For this review, take the finished solid that the model builds, in its own axes (mm). A direction names the side the tool comes from. Round coordinates to 2 decimals unless told otherwise and drop trailing zeros. Order: outer loops, then holes, each group sorted by start corner. A loop starts at its lowest first (then second) coordinate and runs counter-clockwise, first axis right, second up.
from build123d import *

# Parameters (mm, degrees)
F1_DEPTH = 63.5
F0_W     = 4.3192696064
F0_H     = 12.0912648122
F0_H_2   = 11.3655438513
F0_H_3   = 5.1181913365
F2_DEPTH = 25.4
F3_DEPTH = 7.9375
F5_R     = 6.35


with BuildPart() as f1:
    # F0 (on Front) → F1 (new body, symmetric)
    with BuildSketch(Plane.XZ):
        Polygon((-41.275, -9.525), (41.275, -9.525), (41.275, 9.525), (29.9094561487, 9.525), (-41.275, 9.525), align=None)
    extrude(amount=F1_DEPTH, both=True)

    # F0 (on Front) → F2 (join, symmetric)
    with BuildSketch(Plane.XZ):
        with BuildLine():
            Line((29.9094561487, 9.525), (41.275, 9.525))
            Line((41.275, 9.525), (41.275, 37.4912648122))
            ThreePointArc((41.275, 37.4912648122), (45.9246798487, 48.7165849636), (57.15, 53.3662648122))
            Line((57.15, 53.3662648122), (84.2568697843, 53.3662648122))
            Line((84.2568697843, 53.3662648122), (84.2568697843, 64.7318086635))
            Line((84.2568697843, 64.7318086635), (78.3901438117, 64.7318086635))
            Line((78.3901438117, 64.7318086635), (57.15, 64.7318086635))
            ThreePointArc((57.15, 64.7318086635), (37.8880267196, 56.7532380926), (29.9094561487, 37.4912648122))
            Line((29.9094561487, 37.4912648122), (29.9094561487, 9.525))
        make_face()
        with Locations((86.4165045875, 47.3206324061)):
            Rectangle(F0_W, F0_H)
        with Locations((86.4165045875, 59.0490367378)):
            Rectangle(F0_W, F0_H_2)
        with Locations((86.4165045875, 67.2909043317)):
            Rectangle(F0_W, F0_H_3)
        Polygon((88.5761393907, 69.85), (88.5761393907, 64.7318086635), (88.5761393907, 53.3662648122), (88.5761393907, 41.275), (135.0568697843, 41.275), (135.0568697843, 69.85), align=None)
    extrude(amount=F2_DEPTH, both=True)

    # F0 (on Front) → F3 (join, symmetric)
    with BuildSketch(Plane.XZ):
        with BuildLine():
            add(Edge.make_bspline(
                [(-41.275, 9.525), (-36.5560054779, 38.5108739138), (-31.082380563, 73.5029876232), (78.3901438117, 64.7318086635)],
                knots=[0, 0, 0, 0, 131.7859566353, 131.7859566353, 131.7859566353, 131.7859566353], degree=3))
            Line((-41.275, 9.525), (29.9094561487, 9.525))
            Line((29.9094561487, 9.525), (29.9094561487, 37.4912648122))
            ThreePointArc((29.9094561487, 37.4912648122), (37.8880267196, 56.7532380926), (57.15, 64.7318086635))
            Line((57.15, 64.7318086635), (78.3901438117, 64.7318086635))
        make_face()
    extrude(amount=F3_DEPTH, both=True)

    # F0 (on Front) → F4 (revolve)
    with BuildSketch(Plane.XZ):
        Polygon((88.5761393907, 69.85), (88.5761393907, 64.7318086635), (88.5761393907, 53.3662648122), (88.5761393907, 41.275), (135.0568697843, 41.275), (135.0568697843, 69.85), align=None)
    revolve(axis=Axis((135.0568697843, 0, 55.5625), (0, 0, 1)))

    # F5
    f5_edges = [f1.edges().sort_by_distance(p)[0] for p in [
        (41.275, -63.5, 0),
        (-41.275, -63.5, 0),
        (41.275, 63.5, 0),
        (-41.275, 63.5, 0),
    ]]
    fillet(f5_edges, radius=F5_R)


solid = f1.part
(1) Add section B-B on y = 39.5. Give the boundary of the cut face in (x, z) (3 decimals), plus the area to 3 significant figures.
(2) Tool access review of faces 1 (the face through (134, -1, 41.275)), 2 (the face through (55, 25.4, 54)), 3 (the face through (29.909, -17, 24)): name each direction out of +Z, -Z, +X, -X, +Y, -Y from which nothing blocks a thin tool from reaching the whole face with its end or side.
(3) Clearance check with flat-ended pins moving along their axes: P1, Ø10, axis at y = 12.5, z = 7, coming from the +X side (3 decimals); P2, Ø14, axis at y = 20.5, z = 29.5, coming from the -X side; P3, Ø1.5, axis at x = 144.5, z = 61.5, coming from the +Y side; P4, Ø18, axis at x = 74, z = 30, coming from the +Y side. State where each tip first meets the part, or that it passes through.
(4) Add section C-C on x = 150.5. Give the boundary of the cut face in (y, z) (3 decimals), plus the area to 3 significant figures.
(5) Add section A-A on z = -1. Give the boundary of the cut face in (x, y) (3 decimals).
(6) Draft analysis for pull direction X (two halves, no side actions). For faces 4 (the face through (-39.365, 61.689, -0.133)), 5 (the face through (55, -25.4, 54)), 6 (the face through (71, 0, 53.366)), state which applies: pulls with the +X half, pulls with the -X half, needs draft (parallel to the pull), parting line crosses it, or undercut.
(7) Wall thickness on L1, parallel to Y at x = 25, z = 56; L2, parallel to Z at x = -4.5, y = 31 (3 decimals); L3, parallel to X at y = 26, z = 3 (3 decimals): over which ranges is each line inside the solid? List them lowest first.
(8) Add section D-D on y = -22. Give the boundary of the cut face in (x, z) (3 decimals), plus the area to 4 significant figures.
Here are the results:
1. outline: (-41.275, -9.525) - (41.275, -9.525) - (41.275, 9.525) - (-41.275, 9.525) - close; (110.558, 41.275) - (159.556, 41.275) - (159.556, 69.85) - (110.558, 69.85) - close
1. area: 2,970 mm2
2. face 1: -Z, +X, +Y, -Y
2. face 2: +Z, -X, +Y
2. face 3: +Z, -X, -Y
3. P1: stops at x = 41.275
3. P2: stops at x = 29.91
3. P3: stops at y = 45.66
3. P4: passes through
4. outline: (-43.84, 41.275) - (43.84, 41.275) - (43.84, 69.85) - (-43.84, 69.85) - close
4. area: 2,510 mm2
5. outline: (-41.275, -57.15) arc R6.35 ccw to (-34.925, -63.5) - (34.925, -63.5) arc R6.35 ccw to (41.275, -57.15) - (41.275, 57.15) arc R6.35 ccw to (34.925, 63.5) - (-34.925, 63.5) arc R6.35 ccw to (-41.275, 57.15) - close
6. face 4: pulls with the -X half
6. face 5: needs draft
6. face 6: undercut
7. L1: y = -7.94 to 7.94
7. L2: z = -9.525 to 9.525
7. L3: x = -41.275 to 41.275
8. outline: (-41.275, -9.525) - (41.275, -9.525) - (41.275, 37.491) arc R15.875 cw to (57.15, 53.366) - (84.257, 53.366) - (84.257, 41.275) - (176.001, 41.275) - (176.001, 69.85) - (84.257, 69.85) - (84.257, 64.732) - (57.15, 64.732) arc R27.241 ccw to (29.909, 37.491) - (29.909, 9.525) - (-41.275, 9.525) - close
8. area: 5,205 mm2
